The listing builds one solid part. Answer for the finished solid, in the listing's coordinates (mm). A direction names the side the tool comes from. Coordinates: 2 decimals unless noted, no trailing zeros. Loops run counter-clockwise (first coordinate to the right, second up) from the corner with the lowest first, then second, coordinate; pieces in that order, holes last. Notation, with made-up numbers: M 57,-23 L 112,-23 A32 cw 112,15 Z; hole C -37,6 d1. An arc over 180 degrees is marked long. Return JSON: item names as keys, results as strings. Group by question number.
1. Which of the six approach directions +Z, -Z, +X, -X, +Y, -Y give full straight-line access (tool end or side, diameter ignored) to faces 1 (the face through (0, 1, 30)), 2 (the face through (-5, 1, 26)), 3 (the face through (0, 1.5, 26)), 4 (the face through (0, 0.5, 26)), 5 (the face through (5, 1, 26))?
2. Section A-A (x = 2) is taken. Write down the section's boundary in (y, z).
3. Straight lines are drawn through the part: L1, parallel to Z at x = -1.75, y = 1.6; L2, parallel to X at y = 0.7, z = 26. For each, find the intervals that lie inside material, in ascending order. Write a range as from..to.
4. Given P1, Ø0.8, axis at y = 1, z = 27, coming from the -X side; P2, Ø6.5, axis at x = 0, z = 25, coming from the +Y side; P3, Ø1, axis at x = -6, y = 1.5, coming from the +Z side; P4, Ø1.1, axis at y = 1, z = 25, coming from the +X side, each flat-ended and moving along its own axis, determine where each tip first touches the part or whether it passes through.
5. Section B-B (y = 1.05) is taken. Write down the section's boundary in (x, z), then the cut area to 3 significant figures.
6. Section C-C (x = -7.75) is taken. Write down the section's boundary in (y, z).
```python
from build123d import *

# Parameters (mm, degrees)
SKETCH1_W           = 26
SKETCH1_H           = 60
BOSS_EXTRUDE1_DEPTH = 2
SKETCH9_W           = 8
SKETCH9_H           = 8
CUT_EXTRUDE1_DEPTH  = 2
SKETCH10_W          = 10
SKETCH10_H          = 8
CUT_EXTRUDE2_DEPTH  = 0.5
SKETCH11_W          = 10
SKETCH11_H          = 8
CUT_EXTRUDE3_DEPTH  = 0.5


with BuildPart() as part:
    # Sketch1 → Boss-Extrude1 (new body)
    with BuildSketch(Plane(origin=(0, 0, 0), x_dir=(1, 0, 0), z_dir=(0, 1, 0))):
        Rectangle(SKETCH1_W, SKETCH1_H)
    extrude(amount=BOSS_EXTRUDE1_DEPTH)

    # Sketch9 → Cut-Extrude1 (cut)
    with BuildSketch(Plane(origin=(0, 2, 0), x_dir=(1, 0, 0), z_dir=(0, 1, 0))):
        with Locations((-9, -26)):
            Rectangle(SKETCH9_W, SKETCH9_H)
        with Locations((9, -26)):
            Rectangle(SKETCH9_W, SKETCH9_H)
    extrude(amount=-CUT_EXTRUDE1_DEPTH, mode=Mode.SUBTRACT)

    # Sketch10 → Cut-Extrude2 (cut)
    with BuildSketch(Plane(origin=(0, 2, 0), x_dir=(1, 0, 0), z_dir=(0, 1, 0))):
        with Locations((0, -26)):
            Rectangle(SKETCH10_W, SKETCH10_H)
    extrude(amount=-CUT_EXTRUDE2_DEPTH, mode=Mode.SUBTRACT)

    # Sketch11 → Cut-Extrude3 (cut)
    with BuildSketch(Plane.XZ):
        with Locations((0, 26)):
            Rectangle(SKETCH11_W, SKETCH11_H)
    extrude(amount=-CUT_EXTRUDE3_DEPTH, mode=Mode.SUBTRACT)


solid = part.part
```
Worked out:
{
 "1": {"face 1": "+Z, +X, -X, +Y, -Y", "face 2": "+Z, -X, +Y, -Y", "face 3": "+Z, +X, -X, +Y", "face 4": "+Z, +X, -X, -Y", "face 5": "+Z, +X, +Y, -Y"},
 "2": {"outline": "M 0,-30 L 2,-30 L 2,22 L 1.5,22 L 1.5,30 L 0.5,30 L 0.5,22 L 0,22 Z"},
 "3": {"L1": "-30..22", "L2": "-5..5"},
 "4": {"P1": "x = -5", "P2": "y = 2", "P3": "z = 22", "P4": "x = 5"},
 "5": {"outline": "M -13,-30 L 13,-30 L 13,22 L 5,22 L 5,30 L -5,30 L -5,22 L -13,22 Z", "area": "1,430 mm^2"},
 "6": {"outline": "M 0,-30 L 2,-30 L 2,22 L 0,22 Z"}
}
